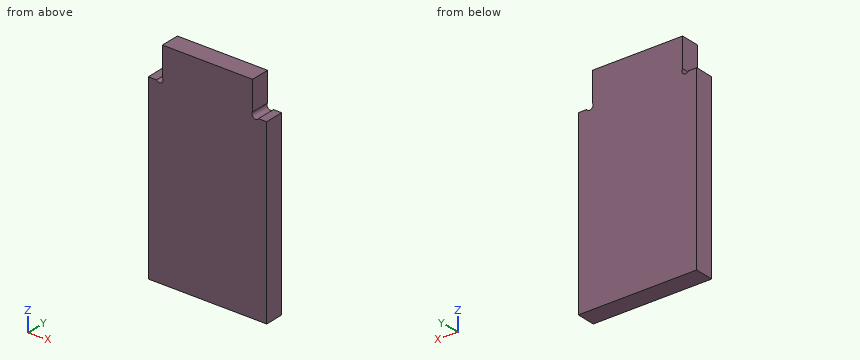
```python
from build123d import *

# Parameters (mm, degrees)
BOSS_EXTRUDE1_DEPTH = 0.4


with BuildPart() as part:
    # Sketch1 → Boss-Extrude1 (new, symmetric)
    with BuildSketch(Plane(origin=(0, 0, 0), x_dir=(1, 0, 0), z_dir=(0, 1, 0))):
        with BuildLine():
            Line((-1.905, -0.167031015), (-1.905, -1.397))
            Line((-1.905, -1.397), (1.905, -1.397))
            Line((1.905, -1.397), (1.905, -0.167031015))
            ThreePointArc((1.905, -0.167031015), (1.946084492, 0.041084492), (2.1542, 0))
            Line((2.1542, 0), (2.5019, 0))
            Line((2.5019, 0), (2.5019, 7.62))
            Line((2.5019, 7.62), (-2.5019, 7.62))
            Line((-2.5019, 7.62), (-2.5019, 0))
            Line((-2.5019, 0), (-2.1542, 0))
            ThreePointArc((-2.1542, 0), (-1.946084492, 0.041084492), (-1.905, -0.167031015))
        make_face()
    extrude(amount=BOSS_EXTRUDE1_DEPTH, both=True)


solid = part.part
```
Geometry check sheet. Reference: the model listing, model coordinates, mm. Round coordinates to 2 decimals unless told otherwise and drop trailing zeros. Loops run counter-clockwise (first coordinate to the right, second up) from the corner with the lowest first, then second, coordinate; pieces in that order, holes last. Notation, with made-up numbers: M -1,68.25 L 32,68.25 A28 ccw 32,87.25 Z; hole C 64.25,25.25 d9. An arc over 180 degrees is marked long. Return JSON: item names as keys, results as strings. Group by question number.
(1) Scan lines: line 1 along X through (y, z) = (0.35, 0.25) (3 decimals); line 2 along Z through (x, y) = (2, -0.1); line 3 along Z through (x, y) = (-2.1, 0.15). Record each from-to range of solid material in increasing order. Write a range as [from, to].
(2) Section check B-B, the plane z = 1. Enter the section's corners in (x, y) (3 decimals), and give its area (3 significant figures).
(3) Section check A-A, the plane y = 0.15. Enter the section's corners in (x, z) (3 decimals), and give its area (3 significant figures).
Data:
{
 "1": {"line 1": "[-1.905, 1.905]", "line 2": "[-7.62, -0.06]", "line 3": "[-7.62, -0.05]"},
 "2": {"outline": "M -1.905,-0.4 L 1.905,-0.4 L 1.905,0.4 L -1.905,0.4 Z", "area": "3.05 mm²"},
 "3": {"outline": "M -2.502,-7.62 L 2.502,-7.62 L 2.502,0 L 2.154,0 A0.15 cw 1.905,0.167 L 1.905,1.397 L -1.905,1.397 L -1.905,0.167 A0.15 cw -2.154,0 L -2.502,0 Z", "area": "43.4 mm²"}
}
